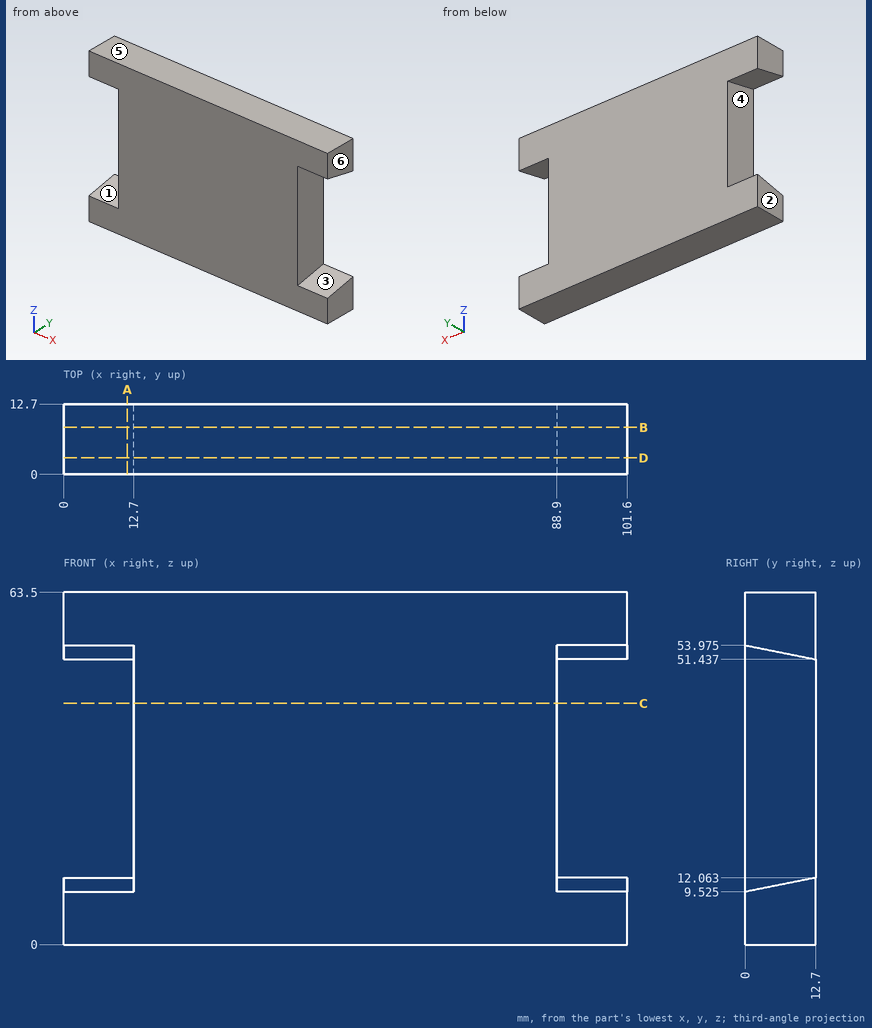
Geometry check sheet. Reference: drawing and pictorial views, mm from the part's lowest x, y, z. A direction names the side the tool comes from. Give positions to 0.01 mm unless a question says otherwise; leave off trailing zeros. Loops run counter-clockwise (first coordinate to the right, second up) from the corner with the lowest first, then second, coordinate; pieces in that order, holes last. Notation, with made-up numbers: (46.5, 78.5) -> (76.5, 78.5) arc R14 cw to (76.5, 103.5) -> close; hole circle Ø7 at (28, 47). An arc over 180 degrees is marked (long way). Answer in a Markdown table with one row per item. Add a question column.
1) Draft check along Z on the marked faces 4, 5 and 6. Enter one of: pulls with the +Z half, pulls with the -Z half, needs draft (parallel to the pull), parting line crosses it, or undercut.
2) Cross-section at C-C on z = 43.5. Record the boundary of the cut face in (x, y), and give its area (3 significant figures).
3) Cross-section at A-A on x = 11.5. Record the boundary of the cut face in (y, z) (1 decimal).
4) Set-up check for the marked faces 1, 2 and 3: record each of +Z, -Z, +X, -X, +Y, -Y from which the full face is reachable in a straight line by a thin tool's end or side.
5) Gauge pin test, flat ends, axial feed: P1, Ø6.5, axis at y = 6.5, z = 34.5, coming from the +X side; P2, Ø1, axis at x = 54.5, z = 55, coming from the -Y side; P3, Ø2, axis at x = 91, z = 37, coming from the -Y side. Record the tip position at first contact, or that the pin passes through.
6) Material ranges on probe 1 along X at (y, z) = (4.5, 29); probe 2 along Z at (x, y) = (10, 5.5), recorded low to high. Write a range as from..to.
7) Cross-section at D-D on y = 3. Record the boundary of the cut face in (x, z) (1 decimal), and give its area (3 significant figures).
8) Cross-section at B-B on y = 8.5. Record the boundary of the cut face in (x, z), and give its area (3 significant figures).
Outcome:
| question | item | result |
|---|---|---|
| 1 | face 4 | undercut |
| 1 | face 5 | pulls with the +Z half |
| 1 | face 6 | needs draft |
| 2 | outline | (12.7, 0) -> (88.9, 0) -> (88.9, 12.7) -> (12.7, 12.7) -> close |
| 2 | area | 968 mm^2 |
| 3 | outline | (0, 0) -> (12.7, 0) -> (12.7, 12.1) -> (0, 9.5) -> close; (0, 54) -> (12.7, 51.4) -> (12.7, 63.5) -> (0, 63.5) -> close |
| 4 | face 1 | -X, -Y |
| 4 | face 2 | +Z, -Z, -X, +Y, -Y |
| 4 | face 3 | +X, -Y |
| 5 | P1 | stops at x = 88.9 |
| 5 | P2 | stops at y = 0 |
| 5 | P3 | passes through |
| 6 | probe 1 | x = 12.7..88.9 |
| 6 | probe 2 | z = 0..10.62, 52.88..63.5 |
| 7 | outline | (0, 0) -> (101.6, 0) -> (101.6, 10.1) -> (88.9, 10.1) -> (88.9, 53.4) -> (101.6, 53.4) -> (101.6, 63.5) -> (0, 63.5) -> (0, 53.4) -> (12.7, 53.4) -> (12.7, 10.1) -> (0, 10.1) -> close |
| 7 | area | 5,350 mm^2 |
| 8 | outline | (0, 0) -> (101.6, 0) -> (101.6, 11.22) -> (88.9, 11.22) -> (88.9, 52.28) -> (101.6, 52.28) -> (101.6, 63.5) -> (0, 63.5) -> (0, 52.28) -> (12.7, 52.28) -> (12.7, 11.22) -> (0, 11.22) -> close |
| 8 | area | 5,410 mm^2 |
